from build123d import *

# Parameters (mm, degrees)
CYLINDER455_R     = 5
CYLINDER455_DEPTH = 100
CYLINDER449_R     = 5
CYLINDER449_DEPTH = 100
CYLINDER457_R     = 5
CYLINDER457_DEPTH = 100
CYLINDER456_R     = 5
CYLINDER456_DEPTH = 100
CYLINDER450_R     = 5
CYLINDER450_DEPTH = 100
CYLINDER458_R     = 5
CYLINDER458_DEPTH = 100
CYLINDER451_R     = 5
CYLINDER451_DEPTH = 100
CYLINDER448_R     = 5
CYLINDER448_DEPTH = 100
BOX197_W          = 10
BOX197_H          = 108
BOX197_DEPTH      = 50
CHAMFER001_SIZE   = 5


with BuildPart() as obj1:
    # Cylinder455 → Cylinder455 (new body)
    with BuildSketch(Plane(origin=(24, -51, 25), x_dir=(0, 0, -1), z_dir=(1, 0, 0))):
        Circle(CYLINDER455_R)
    extrude(amount=CYLINDER455_DEPTH)


with BuildPart() as obj2:
    # Cylinder449 → Cylinder449 (new body)
    with BuildSketch(Plane(origin=(24, 36, 34), x_dir=(0, 0, -1), z_dir=(1, 0, 0))):
        Circle(CYLINDER449_R)
    extrude(amount=CYLINDER449_DEPTH)


with BuildPart() as obj3:
    # Cylinder457 → Cylinder457 (new body)
    with BuildSketch(Plane(origin=(24, -36, 34), x_dir=(0, 0, -1), z_dir=(1, 0, 0))):
        Circle(CYLINDER457_R)
    extrude(amount=CYLINDER457_DEPTH)


with BuildPart() as obj4:
    # Cylinder456 → Cylinder456 (new body)
    with BuildSketch(Plane(origin=(24, -23, -5), x_dir=(0, 0, -1), z_dir=(1, 0, 0))):
        Circle(CYLINDER456_R)
    extrude(amount=CYLINDER456_DEPTH)


with BuildPart() as obj5:
    # Cylinder450 → Cylinder450 (new body)
    with BuildSketch(Plane(origin=(24, 51, 7), x_dir=(0, 0, -1), z_dir=(1, 0, 0))):
        Circle(CYLINDER450_R)
    extrude(amount=CYLINDER450_DEPTH)


with BuildPart() as obj6:
    # Cylinder458 → Cylinder458 (new body)
    with BuildSketch(Plane(origin=(24, 23, -5), x_dir=(0, 0, -1), z_dir=(1, 0, 0))):
        Circle(CYLINDER458_R)
    extrude(amount=CYLINDER458_DEPTH)


with BuildPart() as obj7:
    # Cylinder451 → Cylinder451 (new body)
    with BuildSketch(Plane(origin=(24, -51, 7), x_dir=(0, 0, -1), z_dir=(1, 0, 0))):
        Circle(CYLINDER451_R)
    extrude(amount=CYLINDER451_DEPTH)


with BuildPart() as compound595:
    # Cylinder448 → Cylinder448 (new body)
    with BuildSketch(Plane(origin=(24, 51, 25), x_dir=(0, 0, -1), z_dir=(1, 0, 0))):
        Circle(CYLINDER448_R)
    extrude(amount=CYLINDER448_DEPTH)

    # Compound595: union obj1, obj2, obj3, obj4, obj5, obj6, obj7
    add(obj1.part)
    add(obj2.part)
    add(obj3.part)
    add(obj4.part)
    add(obj5.part)
    add(obj6.part)
    add(obj7.part)


with BuildPart() as compound595_1:
    # Compound595 placement: moved
    add(compound595.part.moved(Location((32, 0, 0))))


with BuildPart() as cut369:
    # Box197 → Box197 (new body)
    with BuildSketch(Plane(origin=(87, -29, -8), x_dir=(1, 0, 0), z_dir=(0, 0, 1))):
        with Locations((5, 54)):
            Rectangle(BOX197_W, BOX197_H)
    extrude(amount=BOX197_DEPTH)

    # Chamfer001
    chamfer001_edges = [cut369.edges().sort_by_distance(p)[0] for p in [
        (87, 25, 42),
    ]]
    chamfer(chamfer001_edges, length=CHAMFER001_SIZE)


with BuildPart() as cut369_1:
    # Chamfer001 placement: moved
    add(cut369.part.moved(Location((8, 6, 0))))

    # Cut369: cut Compound595
    add(compound595_1.part, mode=Mode.SUBTRACT)


solid = cut369_1.part
Geometry check sheet. Reference: the model listing, model coordinates, mm. Round coordinates to 2 decimals unless told otherwise and drop trailing zeros. Write each loop counter-clockwise with the first axis right and the second up, starting at its lowest first coordinate (ties: lowest second). Pieces come first, ordered by that corner, then holes. Notation, with made-up numbers: (7.25, 39) -> (38.25, 39) arc R10 cw to (38.25, 57) -> close; hole circle Ø5 at (52.5, 29). An arc over 180 degrees is marked (long way). One line per item, written item: value. Start each with the question number.
(1) Cross-section at C-C, the plane y = 51. Record the cut outline in (x, z).
(2) Scan lines: line 1 (Y direction, x = 102, z = 34); line 2 (Y direction, x = 98.5, z = 7); line 3 (Z direction, x = 98.5, y = 51). Record each from-to range of solid material in increasing order. Write a range as [from, to].
(3) Cross-section at A-A, the plane z = 25. Record the cut outline in (x, y), and give its area (3 significant figures).
(4) Cross-section at D-D, the plane y = 36. Record the cut outline in (x, z).
(5) Cross-section at B-B, the plane x = 98.75. Record the cut outline in (y, z).
(6) Draft check along Y on faces 1 (the flat face through (98, 30, 40)), 2 (the cylindrical face through (99.93, 37.5, 29.23)), 3 (the cylindrical face through (99.93, -18.494, -2.834)). Enter one of: +Y half, -Y half, draft (parallel to the pull), parting line (faces both ways), or undercut.
(7) Go/stop test with flat-tipped pins: pin 1 Ø3 at (y, z) = (49, 25) entering from +X; pin 2 Ø1 at (x, y) = (99, 52) entering from +Z. Record where each tip stops, or that it passes through.
Answer:
1. outline: (95, -8) -> (105, -8) -> (105, 2) -> (95, 2) -> close; (95, 12) -> (105, 12) -> (105, 20) -> (95, 20) -> close; (95, 30) -> (105, 30) -> (105, 42) -> (100, 42) -> (95, 37) -> close
2. line 1: [-23, 31], [41, 85]
2. line 2: [-23, 46], [56, 85]
2. line 3: [-8, 2], [12, 20], [30, 40.5]
3. outline: (95, -23) -> (105, -23) -> (105, 46) -> (95, 46) -> close; (95, 56) -> (105, 56) -> (105, 85) -> (95, 85) -> close
3. area: 980 mm²
4. outline: (95, -8) -> (105, -8) -> (105, 29) -> (95, 29) -> close; (97, 39) -> (105, 39) -> (105, 42) -> (100, 42) -> close
5. outline: (-23, 0) arc R5 cw to (-19, -8) -> (19, -8) arc R5 cw (long way) to (27, -8) -> (85, -8) -> (85, 40.75) -> (-23, 40.75) -> close; hole circle Ø10 at (36, 34); hole circle Ø10 at (51, 7); hole circle Ø10 at (51, 25)
6. face 1: draft
6. face 2: undercut
6. face 3: -Y half
7. pin 1: through
7. pin 2: z = 41.5
